Study the drawing (mm; zero at the part's minimum x, y, z) and answer. A direction names the side the tool comes from. Coordinates: 2 decimals unless noted, no trailing zeros. Loops run counter-clockwise (first coordinate to the right, second up) from the corner with the lowest first, then second, coordinate; pieces in that order, holes last. Notation, with made-up numbers: (5.25, 19.5) - (20.25, 19.5) arc R14 cw to (20.25, 25.5) - close; hole circle Ø9 at (-8, 6). An arc over 180 degrees is marked (long way). Write each question's results on one line, items separated by ' | '. Start each with the question number.
(1) Find section B-B on y = 2.5. Determine the outline of the cut face in (x, z), then the cut area to 3 significant figures.
(2) Consider line 1 (Z direction, x = 3.25, y = 1.95); line 2 (X direction, y = 2.8, z = 2); line 3 (Z direction, x = 4.75, y = 3.5). Determine where each line is inside the solid, lowest interval first. Write a range as from..to.
(3) For the marked faces 1 and 2, determine the directions among +Z, -Z, +X, -X, +Y, -Y from which every point of the face is accessible in a straight line to the end or side of a thin tool.
(4) Determine the mould class of the marked faces 3, 4 and 5 for opening direction Z: released by +Z, released by -Z, zero draft, split by the parting line, or undercut.
(5) Find section D-D on z = 26.5. Determine the outline of the cut face in (x, y), then the cut area to 3 significant figures.
(6) Find section A-A on x = 9.25. Determine the outline of the cut face in (y, z), then the cut area to 3 significant figures.
(7) Given pin 1 Ø2.5 at (x, z) = (2.83, 2) entering from -Y; pin 2 Ø2.5 at (y, z) = (2.5, 19) entering from -X, each flat-ended and moving along its own axis, determine where each tip first touches the part or whether it passes through.
(8) Find section C-C on x = 3.25. Determine the outline of the cut face in (y, z), then the cut area to 3 significant figures.
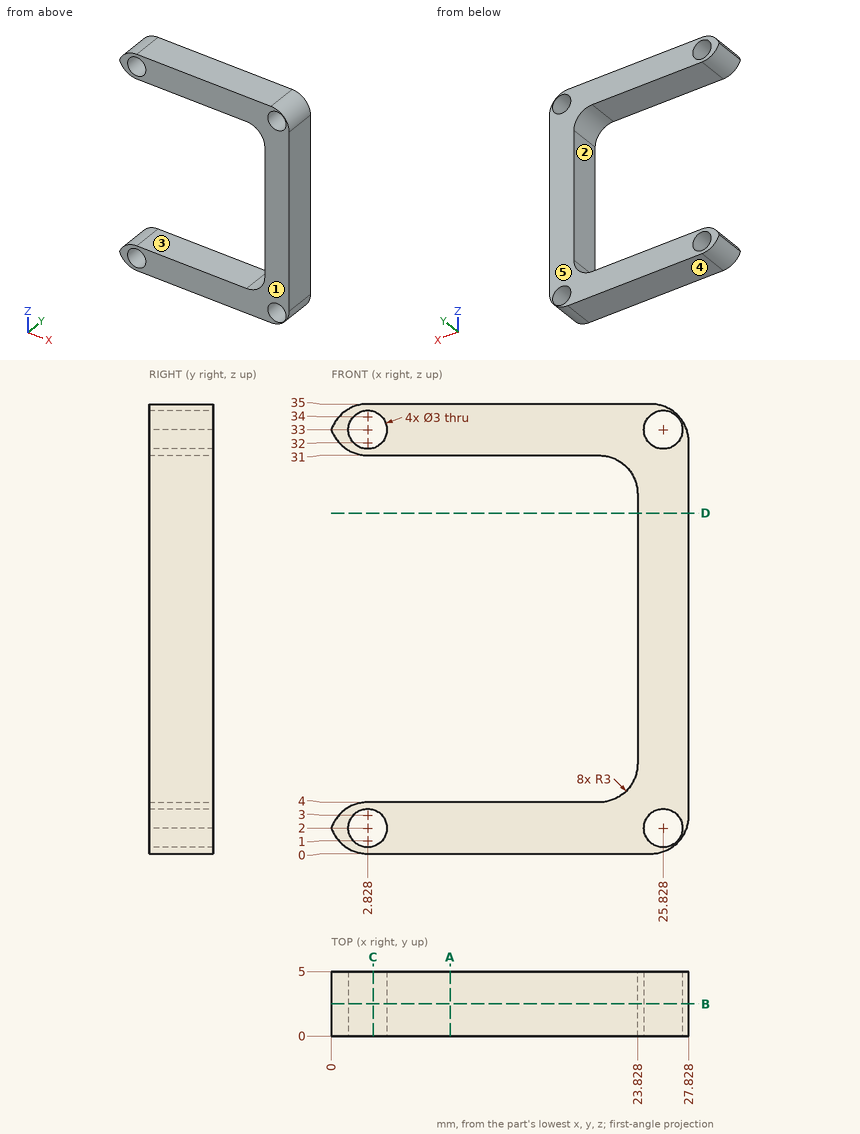
Values:
1) outline: (0, 2) arc R3 ccw to (2.83, 0) - (24.83, 0) arc R3 ccw to (27.83, 3) - (27.83, 32) arc R3 ccw to (24.83, 35) - (2.83, 35) arc R3 ccw to (0, 33) arc R3 ccw to (2.83, 31) - (20.83, 31) arc R3 cw to (23.83, 28) - (23.83, 7) arc R3 cw to (20.83, 4) - (2.83, 4) arc R3 ccw to start; hole circle Ø3 at (2.83, 2); hole circle Ø3 at (2.83, 33); hole circle Ø3 at (25.83, 2); hole circle Ø3 at (25.83, 33) | area: 296 mm²
2) line 1: z = 0..0.56, 3.44..4, 31..31.56, 34.44..35 | line 2: x = 0..1.33, 4.33..24.33, 27.33..27.66 | line 3: z = 0..4, 31..35
3) face 1: +Z, -Z, +X, -X, -Y | face 2: -X, +Y, -Y
4) face 3: undercut | face 4: released by -Z | face 5: zero draft
5) outline: (23.83, 0) - (27.83, 0) - (27.83, 5) - (23.83, 5) - close | area: 20.0 mm²
6) outline: (0, 0) - (5, 0) - (5, 4) - (0, 4) - close; (0, 31) - (5, 31) - (5, 35) - (0, 35) - close | area: 40.0 mm²
7) pin 1: passes through | pin 2: stops at x = 23.83
8) outline: (0, 0) - (5, 0) - (5, 0.56) - (0, 0.56) - close; (0, 3.44) - (5, 3.44) - (5, 4) - (0, 4) - close; (0, 31) - (5, 31) - (5, 31.56) - (0, 31.56) - close; (0, 34.44) - (5, 34.44) - (5, 35) - (0, 35) - close | area: 11.2 mm²
